from build123d import *

# Parameters (mm, degrees)
SKETCH_W      = 48
SKETCH_H      = 50
SKETCH_R      = 1.5
PAD_DEPTH     = 2
SKETCH001_R   = 1.5
PAD001_DEPTH  = 2
SKETCH002_R   = 3.5
SKETCH002_R_2 = 1.5
PAD002_DEPTH  = 2
SKETCH003_R   = 3
SKETCH003_R_2 = 1.5
PAD003_DEPTH  = 4
SKETCH004_R   = 1.5
PAD004_DEPTH  = 7
SKETCH005_R   = 1.5
PAD005_DEPTH  = 7
SKETCH006_R   = 1.5
POCKET_DEPTH  = 5
FILLET_R      = 3
FILLET001_R   = 3
FILLET002_R   = 3
FILLET003_R   = 3


with BuildPart() as body:
    # Sketch → Pad (new body)
    with BuildSketch(Plane.XZ):
        with Locations((24, 25)):
            Rectangle(SKETCH_W, SKETCH_H)
        with Locations((4, 44)):
            Circle(SKETCH_R, mode=Mode.SUBTRACT)
        with Locations((44, 44)):
            Circle(SKETCH_R, mode=Mode.SUBTRACT)
        with Locations((4, 6)):
            Circle(SKETCH_R, mode=Mode.SUBTRACT)
        with Locations((44, 6)):
            Circle(SKETCH_R, mode=Mode.SUBTRACT)
    extrude(amount=PAD_DEPTH)

    # Sketch001 (on Face4 of Pad) → Pad001 (join)
    with BuildSketch(Plane(origin=(0, 0, 0), x_dir=(0, 0, -1), z_dir=(-1, 0, 0))):
        with BuildLine():
            Line((-50, 0), (0, 0))
            Line((0, 14), (0, 0))
            ThreePointArc((0, 14), (-0.494828, 16.210929), (-1.884896, 18))
            Line((-1.884896, 18), (-24.070988, 36.313604))
            ThreePointArc((-24.070988, 36.313604), (-24.966073, 36.823191), (-25.980762, 37))
            Line((-25.980762, 37), (-35.980762, 37))
            ThreePointArc((-35.980762, 37), (-37.468289, 36.605238), (-38.564336, 35.524843))
            Line((-38.564336, 35.524843), (-48.907622, 18))
            ThreePointArc((-48.907622, 18), (-49.721995, 16.07324), (-50, 14))
            Line((-50, 14), (-50, 0))
        make_face()
        with Locations((-5, 14)):
            Circle(SKETCH001_R, mode=Mode.SUBTRACT)
        with Locations((-30.980762, 29)):
            Circle(SKETCH001_R, mode=Mode.SUBTRACT)
        with Locations((-25.980762, 24)):
            Circle(SKETCH001_R, mode=Mode.SUBTRACT)
        with Locations((-25.980762, 34)):
            Circle(SKETCH001_R, mode=Mode.SUBTRACT)
        with Locations((-35.980762, 34)):
            Circle(SKETCH001_R, mode=Mode.SUBTRACT)
        with Locations((-35.980762, 24)):
            Circle(SKETCH001_R, mode=Mode.SUBTRACT)
    extrude(amount=PAD001_DEPTH)

    # Sketch002 (on Face3 of Pad001) → Pad002 (join)
    with BuildSketch(Plane(origin=(48, 0, 0), x_dir=(0, 0, 1), z_dir=(1, 0, 0))):
        with BuildLine():
            Line((24.070988, 36.313604), (1.884896, 18))
            ThreePointArc((1.884896, 18), (0.494828, 16.210929), (0, 14))
            Line((0, 14), (0, 0))
            Line((50, 0), (0, 0))
            Line((50, 14), (50, 0))
            ThreePointArc((50, 14), (49.721995, 16.07324), (48.907622, 18))
            Line((38.564336, 35.524843), (48.907622, 18))
            ThreePointArc((38.564336, 35.524843), (37.468289, 36.605238), (35.980762, 37))
            Line((25.980762, 37), (35.980762, 37))
            ThreePointArc((25.980762, 37), (24.966073, 36.823191), (24.070988, 36.313604))
        make_face()
        with Locations((30.980762, 29)):
            Circle(SKETCH002_R, mode=Mode.SUBTRACT)
        with Locations((5, 14)):
            Circle(SKETCH002_R_2, mode=Mode.SUBTRACT)
    extrude(amount=PAD002_DEPTH)

    # Sketch003 (on Face5 of Pad002) → Pad003 (join)
    with BuildSketch(Plane.XZ.offset(2)):
        with Locations((4, 44)):
            Circle(SKETCH003_R)
        with Locations((4, 44)):
            Circle(SKETCH003_R_2, mode=Mode.SUBTRACT)
        with Locations((44, 44)):
            Circle(SKETCH003_R)
        with Locations((44, 44)):
            Circle(SKETCH003_R_2, mode=Mode.SUBTRACT)
    extrude(amount=PAD003_DEPTH)

    # Sketch004 (on Face8 of Pad003) → Pad004 (join)
    with BuildSketch(Plane(origin=(0, 0, 0), x_dir=(0, 0, 1), z_dir=(1, 0, 0))):
        with BuildLine():
            Line((0, 2), (0, 14))
            ThreePointArc((10, 14), (5, 19), (0, 14))
            Line((10, 14), (10, 2))
            Line((10, 2), (0, 2))
        make_face()
        with Locations((5, 14)):
            Circle(SKETCH004_R, mode=Mode.SUBTRACT)
    extrude(amount=PAD004_DEPTH)

    # Sketch005 (on Face12 of Pad004) → Pad005 (join)
    with BuildSketch(Plane(origin=(48, 0, 0), x_dir=(0, 0, -1), z_dir=(-1, 0, 0))):
        with BuildLine():
            Line((-10, 14), (-10, 2))
            Line((-10, 2), (0, 2))
            Line((0, 2), (0, 14))
            ThreePointArc((0, 14), (-5, 19), (-10, 14))
        make_face()
        with Locations((-5, 14)):
            Circle(SKETCH005_R, mode=Mode.SUBTRACT)
    extrude(amount=PAD005_DEPTH)

    # Sketch006 (on Face6 of Pad005) → Pocket (cut)
    with BuildSketch(Plane.XZ.offset(2)):
        with Locations((4, 6)):
            Circle(SKETCH006_R)
        with Locations((44, 6)):
            Circle(SKETCH006_R)
    extrude(amount=POCKET_DEPTH, mode=Mode.SUBTRACT)

    # Fillet
    fillet_edges = [body.edges().sort_by_distance(p)[0] for p in [
        (48, -2, 30),
    ]]
    fillet(fillet_edges, radius=FILLET_R)

    # Fillet001
    fillet001_edges = [body.edges().sort_by_distance(p)[0] for p in [
        (0, -2, 30),
    ]]
    fillet(fillet001_edges, radius=FILLET001_R)

    # Fillet002
    fillet002_edges = [body.edges().sort_by_distance(p)[0] for p in [
        (7, -2, 5),
    ]]
    fillet(fillet002_edges, radius=FILLET002_R)

    # Fillet003
    fillet003_edges = [body.edges().sort_by_distance(p)[0] for p in [
        (41, -2, 5),
    ]]
    fillet(fillet003_edges, radius=FILLET003_R)


with BuildPart() as part_mirroring:
    # Part__Mirroring: instance of Body
    add(body.part.mirror(Plane(origin=(0, 0, 0), x_dir=(0, -1, 0), z_dir=(1, 0, 0))))


solid = part_mirroring.part
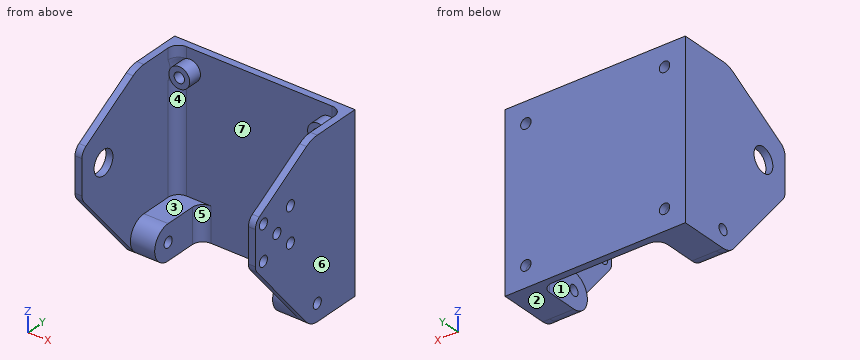
Could you check a few things on this model? Use its own coordinates, in mm. Face numbers are marked on the shaded views. A direction names the side the tool comes from. Give positions to 0.01 mm unless a question says otherwise; leave off trailing zeros. Order: outer loops, then holes, each group sorted by start corner. A loop starts at its lowest first (then second) coordinate and runs counter-clockwise, first axis right, second up.
1. We'd pull the mould along Z, two halves only. Please class the marked faces 1, 2, 3 and 4: pulls with the +Z half, pulls with the -Z half, needs draft (parallel to the pull), parting line crosses it, or undercut.
2. Suppose I cut it at C-C (y = -24). List the corners of the cut face in (x, z) for me.
3. Suppose I cut it at A-A (x = -44). List the corners of the cut face in (y, z) for me, plus the area to 3 significant figures.
4. Suppose I cut it at D-D (z = 14.5). List the corners of the cut face in (x, y) for me, plus the area to 3 significant figures.
5. I need wall thicknesses on L1, parallel to Z at x = -44, y = -3.4; L2, parallel to X at y = -12, z = 13; L3, parallel to Y at x = -3, z = 5. Which ranges of each line are inside material? Lowest first, please.
6. Suppose I cut it at B-B (y = -8.5). List the corners of the cut face in (x, z) for me.
7. For the marked faces 5, 6 and 7, which set-ups out of +Z, -Z, +X, -X, +Y, -Y let a thin tool reach every point of the face, with its end or its side?
8. Will these pins go through, and if not, where does the flat tip stop? P1, Ø8, axis at x = -41.5, y = -29, coming from the +Z side; P2, Ø4, axis at x = -27, z = 41.5, coming from the -Y side; P3, Ø3, axis at x = -40.5, y = -10, coming from the +Z side; P4, Ø1.8, axis at y = -34, z = 35.98, coming from the +X side.
Solved:
1. face 1: needs draft
1. face 2: pulls with the -Z half
1. face 3: undercut
1. face 4: undercut
2. outline: (-50, 9.15) - (-48, 9.15) - (-48, 45.37) - (-50, 45.37) - close; (0, 9.15) - (2, 9.15) - (2, 24.48) - (0, 24.48) - close; (0, 27.48) - (2, 27.48) - (2, 34.48) - (0, 34.48) - close; (0, 37.48) - (2, 37.48) - (2, 45.37) - (0, 45.37) - close
3. outline: (-14, 0) - (0, 0) - (0, 4.5) - (-7, 4.5) - (-7, 7.5) - (0, 7.5) - (0, 42.5) - (-6, 42.5) - (-6, 41) - (-2, 41) - (-2, 10) - (-14, 10) arc R5 ccw to start; (-6, 45.5) - (0, 45.5) - (0, 50) - (-2, 50) - (-2, 47) - (-6, 47) - close; hole circle Ø3 at (-14, 5)
3. area: 237 mm2
4. outline: (-50, -28.41) - (-48, -28.41) - (-48, -5) arc R3 cw to (-45, -2) - (-3, -2) arc R3 cw to (0, -5) - (0, -28.41) - (2, -28.41) - (2, 0) - (-50, 0) - close
4. area: 214 mm2
5. L1: z = 0 to 4.5, 7.5 to 10, 41 to 42.5, 45.5 to 47
5. L2: x = -50 to -48, 0 to 2
5. L3: y = -19 to -15.5, -12.5 to -7
6. outline: (-50, 0) - (-41, 0) - (-41, 10) - (-48, 10) - (-48, 50) - (-50, 50) - close; (-7, 0) - (2, 0) - (2, 50) - (0, 50) - (0, 10) - (-7, 10) - close
7. face 5: +Z, -Z, -Y
7. face 6: +Z, -Z, +X, +Y, -Y
7. face 7: -Y
8. P1: passes through
8. P2: stops at y = -2
8. P3: stops at z = 10
8. P4: stops at x = -48
